Read the model definition and answer for the solid it produces. Units are mm, in the model's axes. Face numbers are marked on the shaded views. A direction names the side the tool comes from. Coordinates: 2 decimals unless noted, no trailing zeros. Loops run counter-clockwise (first coordinate to the right, second up) from the corner with the lowest first, then second, coordinate; pieces in that order, holes last.
from build123d import *

# Parameters (mm, degrees)
SKETCH1_W           = 60
SKETCH1_H           = 60
BOSS_EXTRUDE1_DEPTH = 55
SKETCH2_R           = 18
CUT_EXTRUDE1_DEPTH  = 70.462219947
M5_TAPPED_HOLE1_D   = 4.2
SKETCH5_W           = 45
SKETCH5_H           = 45
CUT_EXTRUDE2_DEPTH  = 14
FILLET1_R           = 5


with BuildPart() as part:
    # Sketch1 → Boss-Extrude1 (new body)
    with BuildSketch(Plane(origin=(0, 0, 0), x_dir=(1, 0, 0), z_dir=(0, 1, 0))):
        Rectangle(SKETCH1_W, SKETCH1_H)
    extrude(amount=BOSS_EXTRUDE1_DEPTH)

    # Sketch2 → Cut-Extrude1 (cut, through all)
    with BuildSketch(Plane(origin=(0, 55, 0), x_dir=(1, 0, 0), z_dir=(0, 1, 0))):
        with Locations(Location((0, 0, 0), (0, 0, 270))):
            Circle(SKETCH2_R)
    extrude(amount=-CUT_EXTRUDE1_DEPTH, mode=Mode.SUBTRACT)

    # M5 Tapped Hole1 (through all)
    with Locations(Plane(origin=(0, 55, 0), x_dir=(1, 0, 0), z_dir=(0, 1, 0))):
        with Locations((-25, -25), (-25, 25), (25, 25), (25, -25), (0, 0)):
            Hole(M5_TAPPED_HOLE1_D / 2)

    # Sketch5 → Cut-Extrude2 (cut)
    with BuildSketch(Plane(origin=(0, 55, 0), x_dir=(1, 0, 0), z_dir=(0, 1, 0))):
        Rectangle(SKETCH5_W, SKETCH5_H)
    extrude(amount=-CUT_EXTRUDE2_DEPTH, mode=Mode.SUBTRACT)

    # Fillet1
    fillet1_edges = [part.edges().sort_by_distance(p)[0] for p in [
        (-22.5, 48, 22.5),
        (-22.5, 48, -22.5),
        (22.5, 48, -22.5),
        (22.5, 48, 22.5),
    ]]
    fillet(fillet1_edges, radius=FILLET1_R)


solid = part.part
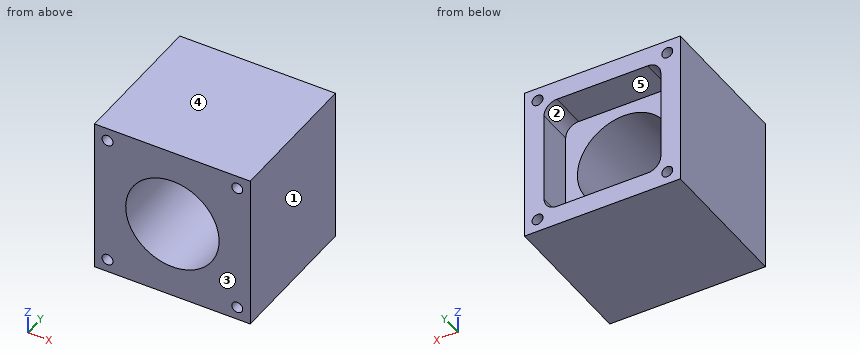
Item 1: A cutting plane is placed at B-B on x = 0. Determine the outline of the cut face in (y, z).
Numbers:
outline: (0, -30) - (55, -30) - (55, -22.5) - (41, -22.5) - (41, -18) - (0, -18) - close; (0, 18) - (41, 18) - (41, 22.5) - (55, 22.5) - (55, 30) - (0, 30) - close
Item 2: A cutting plane is placed at C-C on y = 43. Determine the outline of the cut face in (x, z).
Numbers:
outline: (-30, -30) - (30, -30) - (30, 30) - (-30, 30) - close; hole circle Ø4.2 at (-25, -25); hole circle Ø4.2 at (-25, 25); hole (-22.5, -17.5) arc R5 ccw to (-17.5, -22.5) - (17.5, -22.5) arc R5 ccw to (22.5, -17.5) - (22.5, 17.5) arc R5 ccw to (17.5, 22.5) - (-17.5, 22.5) arc R5 ccw to (-22.5, 17.5) - close; hole circle Ø4.2 at (25, -25); hole circle Ø4.2 at (25, 25)
Item 3: A cutting plane is placed at D-D on z = 0. Determine the outline of the cut face in (x, y).
Numbers:
outline: (-30, 0) - (-18, 0) - (-18, 41) - (-22.5, 41) - (-22.5, 55) - (-30, 55) - close; (18, 0) - (30, 0) - (30, 55) - (22.5, 55) - (22.5, 41) - (18, 41) - close
Item 4: Find the intervals of material crossed by line 1 along X through (y, z) = (22.5, -25); line 2 along X through (y, z) = (31, 0), in increasing order.
Numbers:
line 1: x = -30 to -27.1, -22.9 to 22.9, 27.1 to 30
line 2: x = -30 to -18, 18 to 30
Item 5: Determine the mould class of the marked faces 1, 2 and 3 for opening direction X: released by +X, released by -X, zero draft, split by the parting line, or undercut.
Numbers:
face 1: released by +X
face 2: undercut
face 3: zero draft
Item 6: Which of the six approach directions +Z, -Z, +X, -X, +Y, -Y give full straight-line access (tool end or side, diameter ignored) to the marked faces 4 and 5?
Numbers:
face 4: +Z, +X, -X, +Y, -Y
face 5: +Y
Item 7: A cutting plane is placed at A-A on z = 25. Determine the outline of the cut face in (x, y), then the cut area to 3 significant figures.
Numbers:
outline: (-30, 0) - (-27.1, 0) - (-27.1, 55) - (-30, 55) - close; (-22.9, 0) - (22.9, 0) - (22.9, 55) - (-22.9, 55) - close; (27.1, 0) - (30, 0) - (30, 55) - (27.1, 55) - close
area: 2,840 mm2
